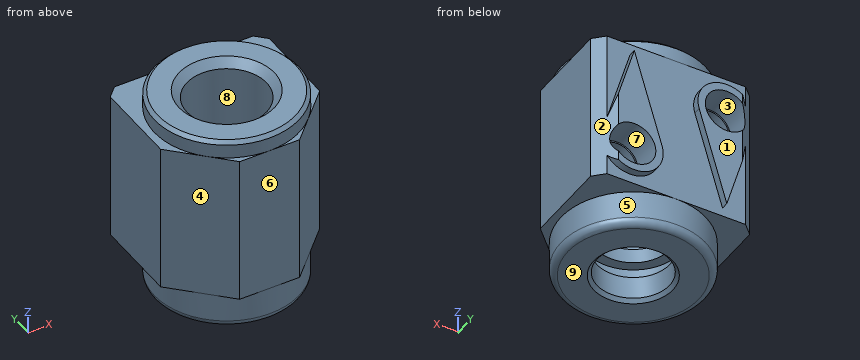
```python
from build123d import *

# Parameters (mm, degrees)
SKETCH1_W                         = 34.925
SKETCH1_H                         = 33.3502
EXTRUDE1_DEPTH                    = 44.45
CUT_EXTRUDE1_DEPTH                = 44.45
SKETCH3_OUTSIDE_W                 = 50.051
SKETCH3_OUTSIDE_H                 = 48.476
SKETCH3_OUTSIDE_R                 = 15.875
CUT_EXTRUDE2_DEPTH                = 3.81
F_1_8_NPT_TAPPED_HOLE1_AT_2_COUNT = 2
F_1_8_NPT_TAPPED_HOLE1_AT_2_PITCH = 25.78600444
SKETCH5_OUTSIDE_W                 = 50.051
SKETCH5_OUTSIDE_H                 = 48.476
SKETCH5_OUTSIDE_R                 = 15.875
CUT_EXTRUDE3_DEPTH                = 7.62
SKETCH6_W                         = 34.925
SKETCH6_H                         = 33.02
CUT_EXTRUDE4_DEPTH                = 1.6002
CUT_EXTRUDE5_DEPTH                = 45.45
F_5_8_0_625_DIAMETER_HOLE1_D      = 15.875
F_3_4_16_TAPPED_HOLE1_D           = 17.526
F_3_4_16_TAPPED_HOLE1_DEPTH       = 25.4
F_3_4_16_TAPPED_HOLE1_TIP         = 5.265341605
SKETCH16_R                        = 10.16
CUT_EXTRUDE7_DEPTH                = 3.556
CHAMFER1_SIZE                     = 0.762
FILLET1_R                         = 1.524
CHAMFER2_SIZE                     = 1.7145
SKETCH18_R                        = 8.763
CUT_EXTRUDE9_DEPTH                = 7.62


with BuildPart() as part:
    # Sketch1 → Extrude1 (new body)
    with BuildSketch(Plane.XY):
        with Locations((17.4625, 16.6751)):
            Rectangle(SKETCH1_W, SKETCH1_H)
    extrude(amount=EXTRUDE1_DEPTH)

    # Sketch2 → Cut-Extrude1 (cut)
    with BuildSketch(Plane.XY.offset(44.45)):
        Polygon((24.038140303, 0), (34.925, 10.886859697), (38.95323648, 7.676224118), (37.650767603, -4.874839611), (-1.660111248, -5.999699096), (-2.784970733, 8.327458557), (0, 10.886859697), (10.886859697, 0), (18.528156354, -3.690776995), align=None)
    extrude(amount=-CUT_EXTRUDE1_DEPTH, mode=Mode.SUBTRACT)

    # Sketch3 outside → Cut-Extrude2 (cut)
    with BuildSketch(Plane.XY.offset(44.45)):
        with Locations((17.4625, 16.675)):
            Rectangle(SKETCH3_OUTSIDE_W, SKETCH3_OUTSIDE_H)
        with Locations((17.4625, 15.875)):
            Circle(SKETCH3_OUTSIDE_R, mode=Mode.SUBTRACT)
    extrude(amount=-CUT_EXTRUDE2_DEPTH, mode=Mode.SUBTRACT)

    # Sketch4 → 1/8 NPT Tapped Hole1 (revolve, cut)
    with BuildSketch(Plane(origin=(7.3025, 33.3502, 31.75), x_dir=(0, 0, 1), z_dir=(1, 0, 0))):
        Polygon((0, 0), (0, 24.377468714), (4.2164, 21.844), (4.2164, 6.35), (4.537409396, 6.35), (4.7275369, 0), align=None)
    f_1_8_npt_tapped_hole1 = revolve(axis=Axis((7.3025, 39.7002, 31.75), (0, -1, 0)), mode=Mode.SUBTRACT)

    # 1/8 NPT Tapped Hole1 at 2: 1/8 NPT Tapped Hole1 ×2
    with Locations(*[Vector(0.788024374, 0, -0.615644042) * (i * F_1_8_NPT_TAPPED_HOLE1_AT_2_PITCH) for i in range(1, F_1_8_NPT_TAPPED_HOLE1_AT_2_COUNT)]):
        add(f_1_8_npt_tapped_hole1, mode=Mode.SUBTRACT)

    # Sketch5 outside → Cut-Extrude3 (cut)
    with BuildSketch(Plane(origin=(0, 0, 0), x_dir=(-1, 0, 0), z_dir=(0, 0, -1))):
        with Locations((-17.4625, 16.675)):
            Rectangle(SKETCH5_OUTSIDE_W, SKETCH5_OUTSIDE_H)
        with Locations(Location((-17.4625, 15.875, 0), (0, 0, 180))):  # turned: the seam where the file's is
            Circle(SKETCH5_OUTSIDE_R, mode=Mode.SUBTRACT)
    extrude(amount=-CUT_EXTRUDE3_DEPTH, mode=Mode.SUBTRACT)

    # Sketch6 → Cut-Extrude4 (cut)
    with BuildSketch(Plane(origin=(0, 33.3502, 0), x_dir=(-1, 0, 0), z_dir=(0, 1, 0))):
        with Locations((-17.4625, 24.13)):
            Rectangle(SKETCH6_W, SKETCH6_H)
        with BuildLine():
            Line((-33.707799282, 17.689285714), (-27.6225, 38.1))
            Line((-27.6225, 38.1), (-21.537200718, 17.689285714))
            ThreePointArc((-21.537200718, 17.689285714), (-27.6225, 9.525), (-33.707799282, 17.689285714))
        make_face(mode=Mode.SUBTRACT)
        with BuildLine():
            Line((-7.3025, 9.525), (-13.387799282, 29.935714286))
            ThreePointArc((-13.387799282, 29.935714286), (-7.839432762, 38.077258744), (-0.998497845, 30.98707351))
            ThreePointArc((-0.998497845, 30.98707351), (-1.209886072, 29.96043147), (-1.587281519, 28.982550324))
            Line((-1.587281519, 28.982550324), (-7.3025, 9.525))
        make_face(mode=Mode.SUBTRACT)
    extrude(amount=-CUT_EXTRUDE4_DEPTH, mode=Mode.SUBTRACT)

    # Sketch8 → Cut-Extrude5 (cut, through all)
    with BuildSketch(Plane.XY.offset(44.45)):
        Polygon((0, 29.5148), (8.827956785, 38.342756785), (29.988545511, 34.451254489), (34.925, 29.5148), (37.769173864, 38.094844764), (-2.725767603, 41.455222953), (-4.620267788, 29.436987401), align=None)
    extrude(amount=-CUT_EXTRUDE5_DEPTH, mode=Mode.SUBTRACT)

    # 5/8 (0.625) Diameter Hole1 (through all)
    with Locations(Plane(origin=(17.4625, 15.875, 44.45), x_dir=(1, 0, 0), z_dir=(0, 0, 1))):
        with Locations((0, 0)):
            Hole(F_5_8_0_625_DIAMETER_HOLE1_D / 2)

    # 3/4-16 Tapped Hole1
    with Locations(Plane(origin=(17.4625, 15.875, 44.45), x_dir=(1, 0, 0), z_dir=(0, 0, 1))):
        with Locations((0, 0)):
            Hole(F_3_4_16_TAPPED_HOLE1_D / 2, depth=F_3_4_16_TAPPED_HOLE1_DEPTH)
            with Locations((0, 0, -(F_3_4_16_TAPPED_HOLE1_DEPTH + F_3_4_16_TAPPED_HOLE1_TIP / 2))):  # 118° drill point
                Cone(0, F_3_4_16_TAPPED_HOLE1_D / 2, F_3_4_16_TAPPED_HOLE1_TIP, mode=Mode.SUBTRACT)

    # Sketch16 → Cut-Extrude7 (cut)
    with BuildSketch(Plane(origin=(0, 0, 5.715), x_dir=(-1, 0, 0), z_dir=(0, 0, -1))):
        with Locations((-17.4625, 15.875)):
            Circle(SKETCH16_R)
    extrude(amount=-CUT_EXTRUDE7_DEPTH, mode=Mode.SUBTRACT)

    # Chamfer1
    chamfer1_edges = [part.edges().sort_by_distance(p)[0] for p in [
        (25.4, 15.875, 0),
        (1.5875, 15.875, 44.45),
    ]]
    chamfer(chamfer1_edges, length=CHAMFER1_SIZE)

    # Fillet1
    fillet1_edges = [part.edges().sort_by_distance(p)[0] for p in [
        (1.5875, 15.875, 0),
    ]]
    fillet(fillet1_edges, radius=FILLET1_R)

    # Chamfer2
    chamfer2_edges = [part.edges().sort_by_distance(p)[0] for p in [
        (26.2255, 15.875, 44.45),
    ]]
    chamfer(chamfer2_edges, length=CHAMFER2_SIZE)

    # Sketch18 → Cut-Extrude9 (cut)
    with BuildSketch(Plane(origin=(0, 0, 12.446), x_dir=(-1, 0, 0), z_dir=(0, 0, -1))):
        with Locations(Location((-17.4625, 15.875, 0), (0, 0, 208.426476552))):  # turned: the seam where the file's is
            Circle(SKETCH18_R)
    extrude(amount=-CUT_EXTRUDE9_DEPTH, mode=Mode.SUBTRACT)


solid = part.part
```
The model under review builds one solid part; all positions refer to its coordinate system, in mm. Face numbers are marked on the shaded views. A direction names the side the tool comes from. Round coordinates to 2 decimals unless told otherwise and drop trailing zeros. Use CSV: the item, a comma, the result in double quotes. Start each with the question number.
(1) Clearance check with flat-ended pins moving along their axes: P1, Ø8, axis at x = 13, y = 16.5, coming from the +Z side; P2, Ø1.5, axis at y = 4.5, z = 21, coming from the -X side; P3, Ø5, axis at x = 7.3, z = 31.75, coming from the +Y side. State where each tip first meets the part, or that it passes through.
(2) Tool access review of the marked faces 5, 6, 7, 8 and 9: name each direction out of +Z, -Z, +X, -X, +Y, -Y from which nothing blocks a thin tool from reaching the whole face with its end or side.
(3) The part is to be moulded in two halves that separate along X. For the marked faces 1, 2, 3 and 4, say which applies: +X half, -X half, draft (parallel to the pull), parting line (faces both ways), or undercut.
(4) For line 1 along Z through (x, y) = (13, 24.5) (3 decimals); line 2 along Z through (x, y) = (27.5, 16.5) (3 decimals); line 3 along Z through (x, y) = (25.5, 21) (3 decimals), list the stretches that pass through material, from the lowest coordinate up.
Findings:
1,P1,"z = 12.45"
1,P2,"x = 5.64"
1,P3,"y = 10.48"
2,face 5,"-Z"
2,face 6,"+Z, -Z, +X, -X, -Y"
2,face 7,"+Y"
2,face 8,"+Z"
2,face 9,"-Z, +X, -X, +Y, -Y"
3,face 1,"draft"
3,face 2,"+X half"
3,face 3,"undercut"
3,face 4,"-X half"
4,line 1,"0 to 5.715, 9.271 to 43.684"
4,line 2,"0 to 5.715, 9.271 to 11.66, 20.09 to 44.029"
4,line 3,"0 to 5.715, 9.271 to 12.232, 19.518 to 43.505"
